Here's how the part is built. I have some questions about the finished solid (model axes, mm). A direction names the side the tool comes from. Give positions to 0.01 mm unless a question says otherwise; leave off trailing zeros. Write each loop counter-clockwise with the first axis right and the second up, starting at its lowest first coordinate (ties: lowest second). Pieces come first, ordered by that corner, then holes. Notation, with made-up numbers: (-29.75, 36) -> (20.25, 36) arc R6 ccw to (20.25, 41) -> close; hole circle Ø5 at (40, 34). An arc over 180 degrees is marked (long way). Answer as CSV lines item,"result". Start each with the question number.
from build123d import *

# Parameters (mm, degrees)
F1_DEPTH = 67.31


with BuildPart() as f1:
    # F0 (on Top) → F1 (new body)
    with BuildSketch(Plane.XY):
        with BuildLine():
            Line((-156.0593098402, -104.9341335893), (117.7671849728, -104.9341335893))
            Line((117.7671849728, -104.9341335893), (117.7671849728, 109.7960919142))
            Line((117.7671849728, 109.7960919142), (-24.6576875478, 109.7960919142))
            ThreePointArc((-24.6576875478, 109.7960919142), (-63.1443316583, 16.8811137323), (-156.0593098402, -21.6055303782))
            Line((-156.0593098402, -21.6055303782), (-156.0593098402, -104.9341335893))
        make_face()
        with BuildLine():
            ThreePointArc((-24.6576875478, 109.7960919142), (-248.9742880221, 202.7110700961), (-156.0593098402, -21.6055303782))
            Line((-156.0593098402, -21.6055303782), (-156.0593098402, 109.7960919142))
            Line((-156.0593098402, 109.7960919142), (-24.6576875478, 109.7960919142))
        make_face()
        with BuildLine():
            Line((-156.0593098402, 109.7960919142), (-156.0593098402, -21.6055303782))
            ThreePointArc((-156.0593098402, -21.6055303782), (-63.1443316583, 16.8811137323), (-24.6576875478, 109.7960919142))
            Line((-24.6576875478, 109.7960919142), (-156.0593098402, 109.7960919142))
        make_face()
    extrude(amount=-F1_DEPTH)


solid = f1.part
Item 1: I'm going to push flat-ended pins straight in: pin 1 (20 mm diameter, centred on y = -79.5, z = -31.5, fed in from -X); pin 2 (10 mm diameter, centred on x = 56, z = -20.5, fed in from +Y); pin 3 (1 mm diameter, centred on y = 198, z = -33, fed in from +X); pin 4 (12 mm diameter, centred on x = -61.5, y = -55, fed in from +Z). Where does each tip first touch, or does it pass through?
Item 2: If we section it at A-A (y = -83.5): Please give me the cut outline in (x, z), and give its area (3 significant figures).
Item 3: If we section it at B-B (z = -42.5): Please give me the cut outline in (x, y), and give its area (3 significant figures).
Item 4: If I drill on line 1 (X direction, y = -69.5, z = -23.5); line 2 (Y direction, x = 100, z = -57); line 3 (Y direction, x = -156, z = -30.5), over which ranges is the centre line in solid material (lowest first)? Write a range as [from, to].
Item 5: If we section it at C-C (x = 40.5): Please give me the cut outline in (y, z), and give its area (3 significant figures).
Item 6: For faces 1 (the face through (48, 109.796, -33)), 2 (the face through (-156.059, -63, -33)), 3 (the face through (-88, 71, 0)), which set-ups out of +Z, -Z, +X, -X, +Y, -Y let a thin tool reach every point of the face, with its end or its side?
Final values:
1,pin 1,"x = -156.06"
1,pin 2,"y = 109.8"
1,pin 3,"x = -58.21"
1,pin 4,"z = 0"
2,outline,"(-156.06, -67.31) -> (117.77, -67.31) -> (117.77, 0) -> (-156.06, 0) -> close"
2,area,"18,400 mm2"
3,outline,"(-156.06, -104.93) -> (117.77, -104.93) -> (117.77, 109.8) -> (-24.66, 109.8) arc R131.4 ccw (long way) to (-156.06, -21.61) -> close"
3,area,"99,500 mm2"
4,line 1,"[-156.06, 117.77]"
4,line 2,"[-104.93, 109.8]"
4,line 3,"[-104.93, 241.2]"
5,outline,"(-104.93, -67.31) -> (109.8, -67.31) -> (109.8, 0) -> (-104.93, 0) -> close"
5,area,"14,500 mm2"
6,face 1,"+Z, -Z, +X, +Y"
6,face 2,"+Z, -Z, -X, -Y"
6,face 3,"+Z, +X, -X, +Y, -Y"
